For this review, take the finished solid that the model builds, in its own axes (mm). A direction names the side the tool comes from. Coordinates: 2 decimals unless noted, no trailing zeros. Loops run counter-clockwise (first coordinate to the right, second up) from the corner with the lowest first, then second, coordinate; pieces in that order, holes last. Notation, with made-up numbers: M 78,29 L 98,29 A19 ccw 98,36 Z; hole C 30.5,21.25 d1. An arc over 180 degrees is marked long. Write each question's results on one line, items separated by ' | '. Start each with the question number.
```python
from build123d import *

# Parameters (mm, degrees)
SKETCH1_W                       = 13.4025
SKETCH1_H                       = 27.8791
CBORE_FOR_M3_SBHCS1_D           = 3.4
CBORE_FOR_M3_SBHCS1_CBORE_D     = 6.7
CBORE_FOR_M3_SBHCS1_CBORE_DEPTH = 2.15
F_10_CLEARANCE_HOLE1_D          = 5.1054


with BuildPart() as part:
    # Sketch1 → Revolve1 (revolve)
    with BuildSketch(Plane.XY, mode=Mode.PRIVATE) as revolve1_sk:
        with Locations((20.98875, 13.93955)):
            Rectangle(SKETCH1_W, SKETCH1_H)
    revolve(revolve1_sk.sketch.rotate(Axis((0, 0, 0), (0, 1, 0)), 90), axis=Axis((0, 0, 0), (0, 1, 0)))

    # CBORE for M3 SBHCS1 (through all)
    with Locations(Plane.XZ):
        with Locations((0, 22.5), (0, -22.5), (22.5, 0), (-22.5, 0)):
            CounterBoreHole(CBORE_FOR_M3_SBHCS1_D / 2, CBORE_FOR_M3_SBHCS1_CBORE_D / 2, CBORE_FOR_M3_SBHCS1_CBORE_DEPTH)

    # #10 Clearance Hole1 (through all)
    with Locations(Plane.XZ):
        with Locations((-11.90625, 20.622229928), (-11.90625, -20.622229928), (11.90625, -20.622229928), (11.90625, 20.622229928)):
            Hole(F_10_CLEARANCE_HOLE1_D / 2)


solid = part.part
```
Q1. Take a section at A-A, the plane z = 0. Give the boundary of the cut face in (x, y).
Q2. Take a section at B-B, the plane x = -7. Give the boundary of the cut face in (y, z), then the cut area to 3 significant figures.
Q3. Take a section at C-C, the plane z = -10.5. Give the boundary of the cut face in (x, y), then the cut area to 3 significant figures.
Q4. For faces 1 (the face through (-25.847, 1.06, 0.147)), 2 (the face through (20.93, 15.19, -0.65)), list the 3-axis set-ups (+Z, -Z, +X, -X, +Y, -Y) from which the entire face can be reached by the end or side of a thin tool; tool diameter is ignored.
Q5. The part is to be moulded in two halves that separate along Z. For faces 3 (the face through (-0.44, 1.06, -19.18)), 4 (the face through (12, 27.879, 12)), 5 (the face through (-0.44, 1.06, 25.82)), 6 (the face through (-8.32, 14.13, -26.41)), say which applies: pulls with the +Z half, pulls with the -Z half, needs draft (parallel to the pull), parting line crosses it, or undercut.
Q6. To check wall thickness, follow line 1 along Z through (x, y) = (-10, 25.25); line 2 along Z through (x, y) = (-12, 5.5); line 3 along Z through (x, y) = (8, 5.75). State the ranges of each line that lie inside material, in increasing order.
Q7. Take a section at D-D, the plane x = -13. Give the boundary of the cut face in (y, z), then the cut area to 3 significant figures.
Q8. Insertion check: P1, Ø4.5, axis at x = 0, z = 22.5, coming from the -Y side; P2, Ø1, axis at x = -10, z = -19.5, coming from the -Y side; P3, Ø12, axis at y = 4, z = 8.5, coming from the -X side; P4, Ø10, axis at y = 3.5, z = 9.5, coming from the +X side. Each pin has a flat end and moves straight along its axis. Give the tip position at first contact, or say it passes through.
Results:
1) outline: M -27.69,0 L -25.85,0 L -25.85,2.15 L -24.2,2.15 L -24.2,27.88 L -27.69,27.88 Z; M -20.8,2.15 L -19.15,2.15 L -19.15,0 L -14.29,0 L -14.29,27.88 L -20.8,27.88 Z; M 14.29,0 L 19.15,0 L 19.15,2.15 L 20.8,2.15 L 20.8,27.88 L 14.29,27.88 Z; M 24.2,2.15 L 25.85,2.15 L 25.85,0 L 27.69,0 L 27.69,27.88 L 24.2,27.88 Z
2) outline: M 0,-26.79 L 27.88,-26.79 L 27.88,-12.46 L 0,-12.46 Z; M 0,12.46 L 27.88,12.46 L 27.88,26.79 L 0,26.79 Z | area: 799 mm^2
3) outline: M -25.62,0 L -9.69,0 L -9.69,27.88 L -25.62,27.88 Z; M 9.69,0 L 25.62,0 L 25.62,27.88 L 9.69,27.88 Z | area: 888 mm^2
4) face 1: -Y | face 2: +Y, -Y
5) face 3: undercut | face 4: needs draft | face 5: undercut | face 6: parting line crosses it
6) line 1: -25.82 to -22.32, -18.92 to -10.2, 10.2 to 18.92, 22.32 to 25.82 | line 2: -24.95 to -23.17, -18.07 to -7.75, 7.75 to 18.07, 23.17 to 24.95 | line 3: -26.51 to -11.84, 11.84 to 26.51
7) outline: M 0,-24.45 L 27.88,-24.45 L 27.88,-22.93 L 0,-22.93 Z; M 0,-18.32 L 27.88,-18.32 L 27.88,-5.93 L 0,-5.93 Z; M 0,5.93 L 27.88,5.93 L 27.88,18.32 L 0,18.32 Z; M 0,22.93 L 27.88,22.93 L 27.88,24.45 L 0,24.45 Z | area: 776 mm^2
8) P1: y = 2.15 | P2: y = 0 | P3: x = -27.58 | P4: x = 27.32
